Read the model definition and answer for the solid it produces. Units are mm, in the model's axes. Face numbers are marked on the shaded views. Round coordinates to 2 decimals unless told otherwise and drop trailing zeros. Write each loop counter-clockwise with the first axis right and the second up, starting at its lowest first coordinate (ties: lowest second). Pieces come first, ordered by that corner, then holes. Notation, with made-up numbers: (27, -2) -> (58, -2) arc R23 cw to (58, 7) -> close; hole circle Ø1 at (20.25, -1). An arc over 180 degrees is marked (long way). Return JSON: item names as keys, results as strings.
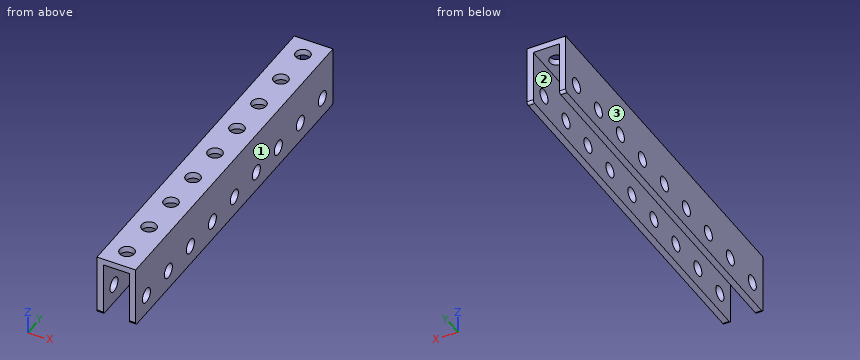
from build123d import *

# Parameters (mm, degrees)
SKETCH1_W                 = 87.757
SKETCH1_H                 = 14.859
BOSS_EXTRUDE1_DEPTH       = 9.398
SKETCH2_W                 = 6.35
SKETCH2_H                 = 13.335
CUT_EXTRUDE1_DEPTH        = 89.888659991
F_5_CLEARANCE_HOLE1_D     = 3.556
F_5_CLEARANCE_HOLE1_DEPTH = 1.524
F_5_CLEARANCE_HOLE2_D     = 3.556
F_5_CLEARANCE_HOLE2_DEPTH = 14.859
F_5_CLEARANCE_HOLE3_D     = 3.556
FILLET1_R                 = 0.635


with BuildPart() as part:
    # Sketch1 → Boss-Extrude1 (new body)
    with BuildSketch(Plane(origin=(-4.699, 0, 0), x_dir=(0, -1, 0), z_dir=(-1, 0, 0))):
        with Locations((-43.8785, -5.9055)):
            Rectangle(SKETCH1_W, SKETCH1_H)
    extrude(amount=-BOSS_EXTRUDE1_DEPTH)

    # Sketch2 → Cut-Extrude1 (cut, through all)
    with BuildSketch(Plane.XZ):
        with Locations((0, -6.6675)):
            Rectangle(SKETCH2_W, SKETCH2_H)
    extrude(amount=-CUT_EXTRUDE1_DEPTH, mode=Mode.SUBTRACT)

    # #5 Clearance Hole1
    with Locations(Plane(origin=(4.699, 0, 0), x_dir=(0, 0, -1), z_dir=(1, 0, 0))):
        with Locations((8.5725, 73.2155), (8.5725, 82.9945), (8.5725, 63.4365), (8.5725, 53.6575), (8.5725, 43.8785), (8.5725, 34.0995), (8.5725, 24.3205), (8.5725, 14.5415), (8.5725, 4.7625)):
            Hole(F_5_CLEARANCE_HOLE1_D / 2, depth=F_5_CLEARANCE_HOLE1_DEPTH)

    # #5 Clearance Hole2
    with Locations(Plane.XY.offset(1.524)):
        with Locations((0, 73.2155), (0, 82.9945), (0, 63.4365), (0, 53.6575), (0, 43.8785), (0, 34.0995), (0, 24.3205), (0, 14.5415), (0, 4.7625)):
            Hole(F_5_CLEARANCE_HOLE2_D / 2, depth=F_5_CLEARANCE_HOLE2_DEPTH)

    # #5 Clearance Hole3 (through all)
    with Locations(Plane(origin=(-3.175, 0, 0), x_dir=(0, 0, -1), z_dir=(1, 0, 0))):
        with Locations((8.5725, 73.2155), (8.5725, 82.9945), (8.5725, 63.4365), (8.5725, 53.6575), (8.5725, 43.8785), (8.5725, 34.0995), (8.5725, 24.3205), (8.5725, 14.5415), (8.5725, 4.7625)):
            Hole(F_5_CLEARANCE_HOLE3_D / 2)

    # Fillet1
    fillet1_edges = [part.edges().sort_by_distance(p)[0] for p in [
        (-3.937, 87.757, -13.335),
        (-3.937, 0, -13.335),
        (3.937, 0, -13.335),
        (3.937, 87.757, -13.335),
    ]]
    fillet(fillet1_edges, radius=FILLET1_R)


solid = part.part
Item 1: Straight lines are drawn through the part: L1, parallel to X at y = 56.5, z = -0.5 (3 decimals); L2, parallel to Z at x = 1.5, y = 22.5. For each, find the intervals that lie inside material, in ascending order. Write a range as [from, to].
Worked answers:
{"L1": "x = [-4.699, -3.175], [3.175, 4.699]", "L2": "z = [0, 1.52]"}
Item 2: Section C-C (x = 0) is taken. State how many separate pieces and enclosed holes the cut face has, then the cut area to 3 significant figures.
Worked answers:
{"separate pieces": "10", "enclosed holes": "0", "area": "85.0 mm2"}
Item 3: Section B-B (y = 70) is taken. Give the vertices of the cut face in (x, z) (3 decimals), then the cut area to 3 significant figures.
Worked answers:
{"outline": "(-4.699, -13.335) -> (-3.175, -13.335) -> (-3.175, 0) -> (3.175, 0) -> (3.175, -13.335) -> (4.699, -13.335) -> (4.699, 1.524) -> (-4.699, 1.524) -> close", "area": "55.0 mm2"}
Item 4: Flat-ended cylindrical pins translate along their axes: pin 1 (2 mm diameter, centred on y = 63.44, z = -8.57, fed in from +X); pin 2 (4 mm diameter, centred on x = 0, y = 53.66, fed in from -Z). Find the tip coordinate at first contact, or state that the pin passes through.
Worked answers:
{"pin 1": "passes through", "pin 2": "stops at z = 0"}
Item 5: For a pull along X with two mould halves and no side action, classify the marked faces 1, 2 and 3 as released by +X, released by -X, zero draft, split by the parting line, or undercut.
Worked answers:
{"face 1": "released by +X", "face 2": "undercut", "face 3": "released by -X"}
Item 6: Section A-A (z = -3.25) is taken. Give the vertices of the cut face in (x, y) (3 decimals), then the cut area to 3 significant figures.
Worked answers:
{"outline": "(-4.699, 0) -> (-3.175, 0) -> (-3.175, 87.757) -> (-4.699, 87.757) -> close; (3.175, 0) -> (4.699, 0) -> (4.699, 87.757) -> (3.175, 87.757) -> close", "area": "267 mm2"}
